Input: part model. Units: mm. Frame: model coordinates. A direction names the side the tool comes from. Coordinates: 2 decimals unless noted, no trailing zeros. Order: outer loops, then holes, each group sorted by start corner. A loop starts at its lowest first (then second) coordinate and runs counter-clockwise, first axis right, second up. Notation, with made-up numbers: (8, 76) - (31, 76) arc R35 cw to (31, 108) - close; hole circle Ø8 at (29, 41.25). An arc over 180 degrees is marked (long way). Use a Markdown table: item, result. Add a question column.
from build123d import *

# Parameters (mm, degrees)
F0_W      = 112.68
F0_H      = 82.6
F0_R      = 1.6
F3_DEPTH  = 1.6
F1_R      = 5
F4_DEPTH  = 1.601
F2_R      = 1.6
F2_R_2    = 3
F2_W      = 2.5
F2_H      = 7
F5_DEPTH  = 1.601
F7_START  = -36.1
F7_DEPTH  = 29
F9_START  = 33
F9_DEPTH  = 32
F1_W      = 10
F1_H      = 1.2
F10_DEPTH = 1.2
F11_SIZE  = 1


with BuildPart() as f3:
    # F0 (on Top) → F3 (new body)
    with BuildSketch(Plane.XY):
        with Locations((56.34, 41.3)):
            Rectangle(F0_W, F0_H)
        with Locations((3.2, 3.2)):
            Circle(F0_R, mode=Mode.SUBTRACT)
        with Locations((94.8, 3.2)):
            Circle(F0_R, mode=Mode.SUBTRACT)
        with Locations((3.2, 79.4)):
            Circle(F0_R, mode=Mode.SUBTRACT)
        with Locations((94.8, 79.4)):
            Circle(F0_R, mode=Mode.SUBTRACT)
    extrude(amount=-F3_DEPTH)

    # F1 (on face) → F4 (cut, through all)
    with BuildSketch(Plane.XY):
        with Locations((80.75, 58.1)):
            Circle(F1_R)
    extrude(amount=-F4_DEPTH, mode=Mode.SUBTRACT)

    # F2 (on face) → F5 (cut, through all)
    with BuildSketch(Plane.XY):
        with Locations((75.75, 4.75)):
            Circle(F2_R)
        with Locations((63, 12)):
            Circle(F2_R_2)
        with Locations((76.25, 12)):
            Rectangle(F2_W, F2_H)
        with Locations((75.75, 19.25)):
            Circle(F2_R)
    extrude(amount=-F5_DEPTH, mode=Mode.SUBTRACT)

    # F6 (on Front) → F7 (join)
    with BuildSketch(Plane.XZ.offset(F7_START)):
        with BuildLine():
            add(Edge.make_bspline(
                [(6.25, 0.9831411553), (6.1998556443, 0.4976120788), (6.25, 0.0696883488), (6.25, 0)],
                knots=[1.5113210061, 1.5113210061, 1.5113210061, 1.5113210061, 2.6925824036, 2.6925824036, 2.6925824036, 2.6925824036], degree=3))
            Line((6.25, 0), (6.25, 0.9831411553))
        make_face()
        with BuildLine():
            Line((5.05, 0), (6.25, 0))
            add(Edge.make_bspline(
                [(6.25, 0.9831411553), (6.1998556443, 0.4976120788), (6.25, 0.0696883488), (6.25, 0)],
                knots=[1.5113210061, 1.5113210061, 1.5113210061, 1.5113210061, 2.6925824036, 2.6925824036, 2.6925824036, 2.6925824036], degree=3))
            Line((6.25, 0.9831411553), (6.25, 3))
            Line((6.25, 3), (5.05, 3))
            Line((5.05, 3), (5.05, 0))
        make_face()
        with BuildLine():
            Line((6.25, 3), (6.25, 0.9831411553))
            add(Edge.make_bspline(
                [(7.25, 2.5), (6.5424729796, 2.3198194624), (6.3141553328, 1.6043332928), (6.25, 0.9831411553)],
                knots=[0, 0, 0, 0, 1.5113210061, 1.5113210061, 1.5113210061, 1.5113210061], degree=3))
            Line((7.25, 2.5), (7.25, 3))
            Line((7.25, 3), (6.25, 3))
        make_face()
        with BuildLine():
            Line((92.05, 0.9831411553), (92.05, 3))
            Line((92.05, 3), (91.05, 3))
            Line((91.05, 3), (91.05, 2.5))
            add(Edge.make_bspline(
                [(91.05, 2.5), (91.7575270204, 2.3198194624), (91.9858446672, 1.6043332928), (92.05, 0.9831411553)],
                knots=[0, 0, 0, 0, 1.5113210061, 1.5113210061, 1.5113210061, 1.5113210061], degree=3))
        make_face()
        with BuildLine():
            Line((93.25, 3), (92.05, 3))
            Line((92.05, 3), (92.05, 0.9831411553))
            add(Edge.make_bspline(
                [(92.05, 0.9831411553), (92.1001443557, 0.4976120788), (92.05, 0.0696883488), (92.05, 0)],
                knots=[1.5113210061, 1.5113210061, 1.5113210061, 1.5113210061, 2.6925824036, 2.6925824036, 2.6925824036, 2.6925824036], degree=3))
            Line((92.05, 0), (93.25, 0))
            Line((93.25, 0), (93.25, 3))
        make_face()
        with BuildLine():
            add(Edge.make_bspline(
                [(92.05, 0.9831411553), (92.1001443557, 0.4976120788), (92.05, 0.0696883488), (92.05, 0)],
                knots=[1.5113210061, 1.5113210061, 1.5113210061, 1.5113210061, 2.6925824036, 2.6925824036, 2.6925824036, 2.6925824036], degree=3))
            Line((92.05, 0.9831411553), (92.05, 0))
        make_face()
    extrude(amount=-F7_DEPTH)

    # F8 (on Right) → F9 (join)
    with BuildSketch(Plane.YZ.offset(F9_START)):
        with BuildLine():
            add(Edge.make_bspline(
                [(80.6190222502, 1.5), (80.7199138112, 0.9911874772), (80.6190222502, 0.2993458475), (80.6190222502, 0)],
                knots=[0.4926390921, 0.4926390921, 0.4926390921, 0.4926390921, 1, 1, 1, 1], degree=3))
            Line((80.6190222502, 0), (81.8190222502, 0))
            Line((81.8190222502, 0), (81.8190222502, 3))
            Line((81.8190222502, 3), (80.6190222502, 3))
            Line((80.6190222502, 3), (80.6190222502, 1.5))
        make_face()
        with BuildLine():
            Line((80.6190222502, 1.5), (80.6190222502, 0))
            add(Edge.make_bspline(
                [(80.6190222502, 1.5), (80.7199138112, 0.9911874772), (80.6190222502, 0.2993458475), (80.6190222502, 0)],
                knots=[0.4926390921, 0.4926390921, 0.4926390921, 0.4926390921, 1, 1, 1, 1], degree=3))
        make_face()
        with BuildLine():
            add(Edge.make_bspline(
                [(79.6190222502, 2.5), (80.2328512073, 2.3155356757), (80.5210582047, 1.9940485863), (80.6190222502, 1.5)],
                knots=[0, 0, 0, 0, 0.4926390921, 0.4926390921, 0.4926390921, 0.4926390921], degree=3))
            Line((80.6190222502, 1.5), (80.6190222502, 3))
            Line((80.6190222502, 3), (79.6190222502, 3))
            Line((79.6190222502, 3), (79.6190222502, 2.5))
        make_face()
    extrude(amount=F9_DEPTH)

    # F1 (on face) → F10 (join)
    with BuildSketch(Plane.XY):
        with Locations((11.25, 21)):
            Rectangle(F1_W, F1_H)
        with Locations((86.75, 21)):
            Rectangle(F1_W, F1_H)
    extrude(amount=F10_DEPTH)

    # F11
    f11_edges = [f3.edges().sort_by_distance(p)[0] for p in [
        (1.6, 79.4, 0),
        (1.6, 3.2, 0),
        (74.15, 4.75, 0),
        (74.15, 19.25, 0),
        (93.2, 3.2, 0),
        (93.2, 79.4, 0),
    ]]
    chamfer(f11_edges, length=F11_SIZE)


solid = f3.part
1) Cut plane B-B (x = 87). Return the cut outline in (y, z), and give its area (3 significant figures).
2) Contact query for flat-ended pins moving along their axis: P1, Ø0.8, axis at y = 50, z = 0.5, coming from the -X side; P2, Ø3, axis at x = 86.5, y = 19.5, coming from the +Z side; P3, Ø0.7, axis at x = 6.5, z = 1.5, coming from the -Y side; P4, Ø3, axis at x = 3.2, y = 3.2, coming from the +Z side. Output: stop coordinate, or through.
3) Pull-direction query (X, two-part tool) for faces 1 (the cylindrical face through (2.85, 77.84, -1.3)), 2 (the flat face through (92, 50, 3)), 3 (the flat face through (5.05, 50, 2)), 4 (the flat face through (93.25, 50, 1)); classes: pulls with the +X half, pulls with the -X half, needs draft (parallel to the pull), parting line crosses it, or undercut.
4) Cut plane C-C (x = 68). Return the cut outline in (y, z), and give its area (3 significant figures).
5) Reachability of faces 5 (the flat face through (92, 36.1, 2)), 6 (the flat face through (6, 65.1, 2)), 7 (the flat face through (65, 81, 2)) from +Z, -Z, +X, -X, +Y, -Y: full face, straight path, thin tool, end or side. Return the list, or none.
6) Material intervals for L1, parallel to Y at x = 3.2, z = -1.4; L2, parallel to X at y = 79.4, z = -1.35; L3, parallel to Y at x = 12, z = 0.5, sorted ascending.
7) Cut plane A-A (y = 19.25). Return the cut outline in (x, z).
Computed:
| question | item | result |
|---|---|---|
| 1 | outline | (0, -1.6) - (82.6, -1.6) - (82.6, 0) - (21.6, 0) - (21.6, 1.2) - (20.4, 1.2) - (20.4, 0) - (0, 0) - close |
| 1 | area | 134 mm2 |
| 2 | P1 | stops at x = 5.05 |
| 2 | P2 | stops at z = 1.2 |
| 2 | P3 | stops at y = 20.4 |
| 2 | P4 | passes through |
| 3 | face 1 | undercut |
| 3 | face 2 | needs draft |
| 3 | face 3 | pulls with the -X half |
| 3 | face 4 | pulls with the +X half |
| 4 | outline | (0, -1.6) - (82.6, -1.6) - (82.6, 0) - (0, 0) - close |
| 4 | area | 132 mm2 |
| 5 | face 5 | +Z, +X, -X, -Y |
| 5 | face 6 | +Z, +X, -X, +Y |
| 5 | face 7 | +Z, +X, +Y, -Y |
| 6 | L1 | y = 0 to 1.6, 4.8 to 77.8, 81 to 82.6 |
| 6 | L2 | x = 0 to 1.6, 4.8 to 93.2, 96.4 to 112.68 |
| 6 | L3 | y = 20.4 to 21.6 |
| 7 | outline | (0, -1.6) - (74.15, -1.6) - (74.15, -1) - (73.15, 0) - (0, 0) - close; (77.35, -1.6) - (112.68, -1.6) - (112.68, 0) - (78.35, 0) - (77.35, -1) - close |
